```python
from build123d import *

# Parameters (mm, degrees)
SKETCH1_W           = 45
SKETCH1_H           = 45
BOSS_EXTRUDE1_DEPTH = 15
FILLET1_R           = 5
SHELL1_T            = -1


with BuildPart() as part:
    # Sketch1 → Boss-Extrude1 (new body)
    with BuildSketch(Plane.XY):
        with Locations((22.5, 22.5)):
            Rectangle(SKETCH1_W, SKETCH1_H)
    extrude(amount=BOSS_EXTRUDE1_DEPTH)

    # Fillet1
    fillet1_edges = [part.edges().sort_by_distance(p)[0] for p in [
        (0, 45, 7.5),
        (45, 45, 7.5),
        (45, 0, 7.5),
        (0, 0, 7.5),
    ]]
    fillet(fillet1_edges, radius=FILLET1_R)

    # Shell1
    shell1_openings = [part.faces().sort_by_distance(p)[0] for p in [
        (22.5, 22.5, 15),
    ]]
    offset(amount=SHELL1_T, openings=shell1_openings, kind=Kind.INTERSECTION)


solid = part.part
```
Here's how the part is built. I have some questions about the finished solid (model axes, mm). A direction names the side the tool comes from. Give positions to 0.01 mm unless a question says otherwise; leave off trailing zeros. Loops run counter-clockwise (first coordinate to the right, second up) from the corner with the lowest first, then second, coordinate; pieces in that order, holes last. Notation, with made-up numbers: M -26.75,14.5 L 15.25,14.5 A19 cw 15.25,50.5 Z; hole C -16.5,9 d8. An arc over 180 degrees is marked long. Put each result on its own line as item: value. Start each with the question number.
(1) I want a section at A-A on z = 10.75. Please give me the cut outline in (x, y).
(2) Will these pins go through, and if not, where does the flat tip stop? pin 1 Ø5 at (x, y) = (39.5, 4.5) entering from -Z; pin 2 Ø1.5 at (x, y) = (12.5, 33.5) entering from +Z.
(3) If we mould it in two halves opening along X, with no side actions, what happens to faces 3 (the flat face through (1, 22, 8)), 4 (the cylindrical face through (1, 2, 8)), 5 (the flat face through (45, 22, 7))? For each: +X half, -X half, draft (parallel to the pull), parting line (faces both ways), or undercut.
(4) For faces 1 (the flat face through (22, 23, 0)), 2 (the cylindrical face through (2.141, 42.797, 8.098)), which set-ups out of +Z, -Z, +X, -X, +Y, -Y let a thin tool reach every point of the face, with its end or its side?
(5) I want a section at B-B on x = 39. Please give me the cut outline in (y, z), then the cut area to 3 significant figures.
(6) I need wall thicknesses on line 1 along Y through (x, z) = (33, 8); line 2 along Z through (x, y) = (27, 25). Which ranges of each line are inside material? Lowest first, please. Write a range as [from, to].
Answer block:
1. outline: M 0,5 A5 ccw 5,0 L 40,0 A5 ccw 45,5 L 45,40 A5 ccw 40,45 L 5,45 A5 ccw 0,40 Z; hole M 1,5 A4 ccw 5,1 L 40,1 A4 ccw 44,5 L 44,40 A4 ccw 40,44 L 5,44 A4 ccw 1,40 Z
2. pin 1: z = 0
2. pin 2: z = 1
3. face 3: undercut
3. face 4: -X half
3. face 5: +X half
4. face 1: -Z, +X, -X, +Y, -Y
4. face 2: +Z
5. outline: M 0,0 L 45,0 L 45,15 L 44,15 L 44,1 L 1,1 L 1,15 L 0,15 Z
5. area: 73.0 mm^2
6. line 1: [0, 1], [44, 45]
6. line 2: [0, 1]
